Input: part model. Units: mm. Frame: model coordinates. A direction names the side the tool comes from. Round coordinates to 2 decimals unless told otherwise and drop trailing zeros. Loops run counter-clockwise (first coordinate to the right, second up) from the corner with the lowest first, then second, coordinate; pieces in that order, holes last. Notation, with made-up numbers: (49.25, 15) -> (108.25, 15) arc R10 cw to (108.25, 24) -> close; hole circle Ø3 at (38.5, 7). An arc over 180 degrees is marked (long way). Answer as a JSON object with one key per item and string values.
```python
from build123d import *

# Parameters (mm, degrees)
SKETCH_1_W          = 21.5
SKETCH_1_H          = 26
EXTRUDE_1_DEPTH     = 12
SKETCH_2_W          = 22.422219076
SKETCH_2_H          = 9.017669608
CUT_EXTRUDE_1_DEPTH = 36.80851854
CHAMFER_1_SIZE      = 2
CHAMFER_2_SIZE      = 4
SKETCH_3_R          = 1.5
CUT_EXTRUDE_2_DEPTH = 36.80851854
SKETCH_4_W          = 13.5
SKETCH_4_H          = 18.032522109
CUT_EXTRUDE_3_DEPTH = 36.80851854
CHAMFER_3_SIZE      = 2


with BuildPart() as part:
    # Эскиз1 → Вытянуть1 (new body)
    with BuildSketch(Plane(origin=(0, 0, 0), x_dir=(1, 0, 0), z_dir=(0, 1, 0))):
        with Locations((10.75, -13)):
            Rectangle(SKETCH_1_W, SKETCH_1_H)
    extrude(amount=EXTRUDE_1_DEPTH)

    # Эскиз2 → Вырез-Вытянуть1 (cut, through all)
    with BuildSketch(Plane(origin=(21.5, 0, 0), x_dir=(0, 0, -1), z_dir=(1, 0, 0))):
        with Locations((-20.227370593, 8.508834804)):
            Rectangle(SKETCH_2_W, SKETCH_2_H)
    extrude(amount=-CUT_EXTRUDE_1_DEPTH, mode=Mode.SUBTRACT)

    # Фаска1
    chamfer_1_edges = [part.edges().sort_by_distance(p)[0] for p in [
        (10.75, 12, 0),
        (10.75, 12, 9.016261055),
    ]]
    chamfer(chamfer_1_edges, length=CHAMFER_1_SIZE)

    # Фаска2
    chamfer_2_edges = [part.edges().sort_by_distance(p)[0] for p in [
        (10.75, 0, 0),
    ]]
    chamfer(chamfer_2_edges, length=CHAMFER_2_SIZE)

    # Эскиз3 → Вырез-Вытянуть2 (cut, through all)
    with BuildSketch(Plane(origin=(21.5, 0, 0), x_dir=(0, 0, -1), z_dir=(1, 0, 0))):
        with Locations((-4.508130527, 7.777054312)):
            Circle(SKETCH_3_R)
    extrude(amount=-CUT_EXTRUDE_2_DEPTH, mode=Mode.SUBTRACT)

    # Эскиз4 → Вырез-Вытянуть3 (cut, through all)
    with BuildSketch(Plane(origin=(0, 12, 0), x_dir=(1, 0, 0), z_dir=(0, 1, 0))):
        with Locations((10.75, -2.983738945)):
            Rectangle(SKETCH_4_W, SKETCH_4_H)
    extrude(amount=-CUT_EXTRUDE_3_DEPTH, mode=Mode.SUBTRACT)

    # Фаска3
    chamfer_3_edges = [part.edges().sort_by_distance(p)[0] for p in [
        (10.75, 0, 26),
    ]]
    chamfer(chamfer_3_edges, length=CHAMFER_3_SIZE)


solid = part.part
```
1) Ray query, probe 1 along X at (y, z) = (9, 2.5); probe 2 along Y at (x, z) = (18.25, 21.5); probe 3 along Z at (x, y) = (8.75, 2.75). Return the intervals inside material, ascending.
Output:
{"probe 1": "x = 0 to 4, 17.5 to 21.5", "probe 2": "y = 0 to 4", "probe 3": "z = 12 to 26"}
2) Reachability of faces 4 (the face through (19, 2, 2)), 5 (the face through (2, 7, 9.016)) from +Z, -Z, +X, -X, +Y, -Y: full face, straight path, thin tool, end or side. Return the list, or none.
Output:
{"face 4": "-Z, +X, -X, -Y", "face 5": "+Z, +X, -X, +Y"}
3) Section C-C, the plane y = 7. Output: boundary loops of the cut face in (x, z), plus the area to 3 significant figures.
Output:
{"outline": "(0, 0) -> (4, 0) -> (4, 3.23) -> (0, 3.23) -> close; (0, 5.79) -> (4, 5.79) -> (4, 9.02) -> (0, 9.02) -> close; (17.5, 0) -> (21.5, 0) -> (21.5, 3.23) -> (17.5, 3.23) -> close; (17.5, 5.79) -> (21.5, 5.79) -> (21.5, 9.02) -> (17.5, 9.02) -> close", "area": "51.6 mm^2"}
4) Draft query along Y for faces 1 (the face through (2.028, 9.264, 4.703)), 2 (the face through (2, 11, 1)), 3 (the face through (20, 7, 9.016)). Return one class per face: +Y half, -Y half, draft (parallel to the pull), parting line (faces both ways), or undercut.
Output:
{"face 1": "undercut", "face 2": "+Y half", "face 3": "draft"}
5) Section B-B, the plane y = 4.5. Output: boundary loops of the cut face in (x, z).
Output:
{"outline": "(0, 0) -> (4, 0) -> (4, 9.02) -> (0, 9.02) -> close; (17.5, 0) -> (21.5, 0) -> (21.5, 9.02) -> (17.5, 9.02) -> close"}
6) Section A-A, the plane z = 11.5. Output: boundary loops of the cut face in (x, y).
Output:
{"outline": "(0, 0) -> (4, 0) -> (4, 4) -> (0, 4) -> close; (17.5, 0) -> (21.5, 0) -> (21.5, 4) -> (17.5, 4) -> close"}
7) Contact query for flat-ended pins moving along their axis: P1, Ø3, axis at x = 3, y = 7.5, coming from the +Z side; P2, Ø8.5, axis at x = 12, z = 14, coming from the +Y side; P3, Ø1.8, axis at y = 7.78, z = 4.51, coming from the -X side; P4, Ø3, axis at x = 12, y = 2, coming from the -Z side. Output: stop coordinate, or through.
Output:
{"P1": "stops at z = 9.02", "P2": "stops at y = 4", "P3": "passes through", "P4": "stops at z = 12"}
8) Section D-D, the plane x = 4.5. Output: boundary loops of the cut face in (y, z).
Output:
{"outline": "(0, 12) -> (4, 12) -> (4, 26) -> (2, 26) -> (0, 24) -> close"}
